Check sheet for the modelled part. Datum: model origin and axes. Units: mm. Face numbers are marked on the shaded views. A direction names the side the tool comes from. Give positions to 0.01 mm unless a question says otherwise; leave off trailing zeros. Write each loop counter-clockwise with the first axis right and the second up, starting at its lowest first coordinate (ties: lowest second). Pieces come first, ordered by that corner, then holes. Notation, with made-up numbers: (17.5, -20) - (47.5, -20) arc R16 cw to (47.5, 1) - close; hole circle Ø2 at (-7.5, 1). An arc over 180 degrees is marked (long way). Return JSON: item names as keys, results as strings. Group by question number.
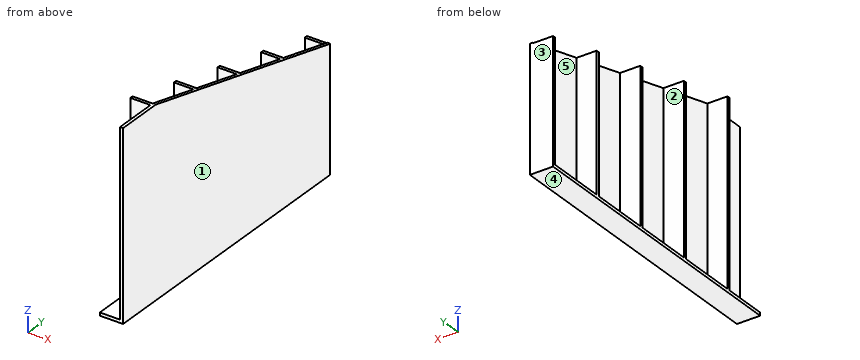
```python
from build123d import *

# Parameters (mm, degrees)
BOSS_EXTRUDE4_DEPTH = 150
BOSS_EXTRUDE5_START = -150
BOSS_EXTRUDE5_DEPTH = 20


with BuildPart() as part:
    # Sketch1 → Boss-Extrude4 (new body)
    with BuildSketch(Plane(origin=(0, 0, 0), x_dir=(0, 0, -1), z_dir=(1, 0, 0))):
        Polygon((-20, 0), (0, 0), (0, 1900), (-800, 1900), (-800, 1880), (-20, 1880), (-20, 1500), (-902.5, 1500), (-902.5, 1480), (-20, 1480), (-20, 1100), (-1002.5, 1100), (-1002.5, 1080), (-20, 1080), (-20, 700), (-1102.5, 700), (-1102.5, 680), (-20, 680), (-20, 300), (-1200, 300), (-1200, 280), (-20, 280), align=None)
    extrude(amount=BOSS_EXTRUDE4_DEPTH)

    # Sketch2 → Boss-Extrude5 (add)
    with BuildSketch(Plane.ZY.offset(BOSS_EXTRUDE5_START)):
        Polygon((0, 1900), (803.333333333, 1900), (1200, 300), (1200, 0), (0, 0), align=None)
    extrude(amount=BOSS_EXTRUDE5_DEPTH)


solid = part.part
```
Item 1: Section check C-C on y = 830.5. Record the cut outline in (x, z).
Item 2: Depth check by flat-ended pin: pin 1 (1.5 mm diameter, centred on x = 108, y = 573.5, fed in from +Z); pin 2 (1.5 mm diameter, centred on x = 55.5, z = 377, fed in from -Y); pin 3 (6 mm diameter, centred on x = 66.5, y = 690.5, fed in from +Z). Enter the tip coordinate at first touch or a pass-through.
Item 3: Material ranges on line 1 along Y through (x, z) = (51.5, 466); line 2 along Y through (x, z) = (27, 845); line 3 along Y through (x, z) = (30, 1014.5), recorded low to high. Write a range as from..to.
Item 4: Mould release check, pull along Y, two halves, no side actions. Record for the marked faces 3, 4 and 5: +Y half, -Y half, draft (parallel to the pull), parting line (faces both ways), or undercut.
Item 5: Access from +Z, -Z, +X, -X, +Y, -Y to the whole of each face (thin tool, end or side, straight path). Record for the marked faces 1 and 2.
Item 6: Section check B-B on x = 57. Record the cut outline in (y, z).
Item 7: Section check D-D on z = 922.5. Record the cut outline in (x, y), plus the area to 3 significant figures.
Item 8: Section check A-A on z = 615.5. Record the cut outline in (x, y), plus the area to 3 significant figures.
Reply:
{
 "1": {"outline": "(0, 0) - (150, 0) - (150, 1068.48) - (130, 1068.48) - (130, 20) - (0, 20) - close"},
 "2": {"pin 1": "z = 20", "pin 2": "y = 280", "pin 3": "z = 1102.5"},
 "3": {"line 1": "280..300, 680..700, 1080..1100, 1480..1500, 1880..1900", "line 2": "280..300, 680..700, 1080..1100, 1480..1500", "line 3": "280..300, 680..700"},
 "4": {"face 3": "+Y half", "face 4": "draft", "face 5": "undercut"},
 "5": {"face 1": "+Z, -Z, +X, +Y, -Y", "face 2": "+Z, -X"},
 "6": {"outline": "(0, 0) - (1900, 0) - (1900, 800) - (1880, 800) - (1880, 20) - (1500, 20) - (1500, 902.5) - (1480, 902.5) - (1480, 20) - (1100, 20) - (1100, 1002.5) - (1080, 1002.5) - (1080, 20) - (700, 20) - (700, 1102.5) - (680, 1102.5) - (680, 20) - (300, 20) - (300, 1200) - (280, 1200) - (280, 20) - (0, 20) - close"},
 "7": {"outline": "(0, 280) - (130, 280) - (130, 0) - (150, 0) - (150, 1419.33) - (130, 1419.33) - (130, 1100) - (0, 1100) - (0, 1080) - (130, 1080) - (130, 700) - (0, 700) - (0, 680) - (130, 680) - (130, 300) - (0, 300) - close", "area": "36,200 mm²"},
 "8": {"outline": "(0, 280) - (130, 280) - (130, 0) - (150, 0) - (150, 1900) - (0, 1900) - (0, 1880) - (130, 1880) - (130, 1500) - (0, 1500) - (0, 1480) - (130, 1480) - (130, 1100) - (0, 1100) - (0, 1080) - (130, 1080) - (130, 700) - (0, 700) - (0, 680) - (130, 680) - (130, 300) - (0, 300) - close", "area": "51,000 mm²"}
}
